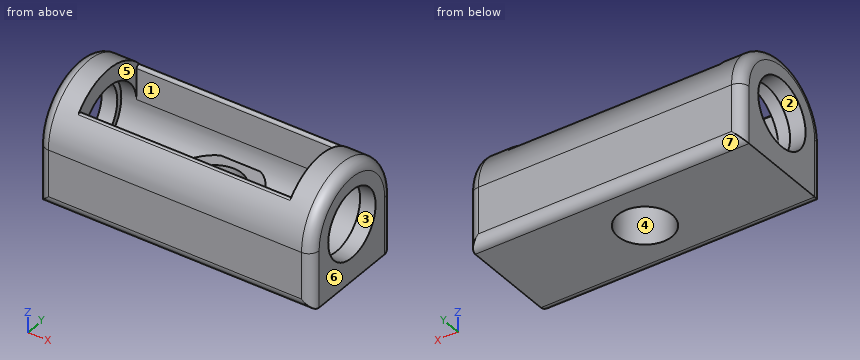
from build123d import *
from build123d.topology import SkipClean

# Parameters (mm, degrees)
BOSS_EXTRUDE1_DEPTH = 26.5
CUT_EXTRUDE2_REACH  = 38.729
CUT_EXTRUDE2_START  = -6
CUT_EXTRUDE3_REACH  = 32.729
SKETCH4_R           = 6.5
CUT_EXTRUDE6_START  = -3
SKETCH7_R           = 7.6000000000000005
CUT_EXTRUDE6_DEPTH  = 3
BOSS_EXTRUDE4_REACH = 60.236
BOSS_EXTRUDE4_START = -3
SKETCH8_R           = 7.999999999999998
CUT_EXTRUDE4_START  = -11
SKETCH5_R           = 5.2499999999999964
CUT_EXTRUDE4_DEPTH  = 8
FILLET1_R           = 2
FILLET2_R           = 0.5


with BuildPart() as part:
    # Sketch1 → Boss-Extrude1 (new body)
    with BuildSketch(Plane(origin=(0, 0, 0), x_dir=(0, 0, -1), z_dir=(1, 0, 0))):
        with BuildLine():
            Line((0, 11), (11.000000000000002, 11))
            Line((11.000000000000002, 11), (11.000000000000002, -11))
            Line((11.000000000000002, -11), (3.47e-15, -11))
            ThreePointArc((3.47e-15, -11), (-11, 1.35e-15), (0, 11))
        make_face()
    boss_extrude1 = extrude(amount=BOSS_EXTRUDE1_DEPTH)

    # Sketch3 → Cut-Extrude2 (cut, up to next)
    with BuildSketch(Plane.ZY.offset(CUT_EXTRUDE2_START), mode=Mode.PRIVATE) as cut_extrude2_sk1:
        with BuildLine():
            Line((0.7418695651929484, 7.5637047502028025), (10.999999999999998, 7.5637047502028025))
            Line((10.999999999999998, 7.5637047502028025), (11, -7.599999999999998))
            Line((11, -7.599999999999998), (9.3e-16, -7.6))
            ThreePointArc((9.3e-16, -7.6), (-7.590920764358606, 0.3713784447559566), (0.7418695651929484, 7.5637047502028025))
        make_face()
    cut_extrude2_tool1 = extrude(cut_extrude2_sk1.sketch, amount=-CUT_EXTRUDE2_REACH, mode=Mode.PRIVATE) & part.part
    cut_extrude2 = cut_extrude2_tool1.solids().sort_by_distance((6, -0.011225, 2.425795))[0]
    add(cut_extrude2, mode=Mode.SUBTRACT)

    # Sketch4 → Cut-Extrude3 (cut, up to next)
    with BuildSketch(Plane.ZY, mode=Mode.PRIVATE) as cut_extrude3_sk1:
        Circle(SKETCH4_R)
    cut_extrude3_tool1 = extrude(cut_extrude3_sk1.sketch, amount=-CUT_EXTRUDE3_REACH, mode=Mode.PRIVATE) & part.part
    cut_extrude3 = cut_extrude3_tool1.solids().sort_by_distance((0, 0, 0))[0]
    add(cut_extrude3, mode=Mode.SUBTRACT)

    # Sketch7 → Cut-Extrude6 (cut)
    with BuildSketch(Plane(origin=(6, 0, 0), x_dir=(0, 0, -1), z_dir=(1, 0, 0)).offset(CUT_EXTRUDE6_START)):
        with Locations(Location((0, 0, 0), (0, 0, 95.601814437))):
            Circle(SKETCH7_R)
    cut_extrude6 = extrude(amount=CUT_EXTRUDE6_DEPTH, mode=Mode.SUBTRACT)

    # Mirror1: Boss-Extrude1, Cut-Extrude2, Cut-Extrude3, Cut-Extrude6 across plane
    with SkipClean():  # the faces are left unmerged after this step: merging them gives an invalid solid
        add(boss_extrude1.mirror(Plane(origin=(26.5, 0, 0), x_dir=(0, 0, 1), z_dir=(1, 0, 0))))
        add(cut_extrude2.mirror(Plane(origin=(26.5, 0, 0), x_dir=(0, 0, 1), z_dir=(1, 0, 0))), mode=Mode.SUBTRACT)
        add(cut_extrude3.mirror(Plane(origin=(26.5, 0, 0), x_dir=(0, 0, 1), z_dir=(1, 0, 0))), mode=Mode.SUBTRACT)
        add(cut_extrude6.mirror(Plane(origin=(26.5, 0, 0), x_dir=(0, 0, 1), z_dir=(1, 0, 0))), mode=Mode.SUBTRACT)

    # Sketch8 → Boss-Extrude4 (add, up to next)
    with BuildSketch(Plane.XY.offset(BOSS_EXTRUDE4_START), mode=Mode.PRIVATE) as boss_extrude4_sk1:
        with Locations((26.499999999999996, 3.1e-16)):
            Circle(SKETCH8_R)
    boss_extrude4_tool1 = extrude(boss_extrude4_sk1.sketch, amount=-BOSS_EXTRUDE4_REACH, mode=Mode.PRIVATE) - part.part
    add(boss_extrude4_tool1.solids().sort_by_distance((26.5, 0, -3))[0])

    # Sketch5 → Cut-Extrude4 (cut)
    with SkipClean():  # the faces are left unmerged after this step: merging them gives an invalid solid
        with BuildSketch(Plane.XY.offset(CUT_EXTRUDE4_START)):
            with Locations((26.499999999999996, 3.1e-16)):
                Circle(SKETCH5_R)
        extrude(amount=CUT_EXTRUDE4_DEPTH, mode=Mode.SUBTRACT)

    # Fillet1
    fillet1_edges = [part.edges().sort_by_distance(p)[0] for p in [
        (53, -11, -5.500000000000003),
        (53, 11, -5.500000000000001),
        (53, -1.7e-15, 11),
        (0, -1.7e-15, 11),
        (0, 11, -5.500000000000001),
        (0, -11, -5.500000000000003),
        (26.5, 11, -11.000000000000002),
        (26.5, -11, -11.000000000000002),
    ]]
    fillet(fillet1_edges, radius=FILLET1_R)

    # Fillet2
    fillet2_edges = [part.edges().sort_by_distance(p)[0] for p in [
        (26.5, -7.599999999999999, 7.9523581408284185),
        (26.5, 7.5637047502028025, 7.9868874069789895),
    ]]
    fillet(fillet2_edges, radius=FILLET2_R)


solid = part.part
Verification items for the finished model (mm, model axes). Face numbers are marked on the shaded views. A direction names the side the tool comes from. Coordinates: 2 decimals unless noted, no trailing zeros. Write each loop counter-clockwise with the first axis right and the second up, starting at its lowest first coordinate (ties: lowest second). Pieces come first, ordered by that corner, then holes. Notation, with made-up numbers: M 74,22.25 L 99,22.25 A18 ccw 99,48.25 Z; hole C -34.75,7.25 d1. An arc over 180 degrees is marked long. One line per question, with ' | ' between items.
1) Sectioned sample at B-B on x = 5.5. Record the cut outline in (y, z).
Solutions:
outline: M -11,-9 A2 ccw -9,-11 L 9,-11 A2 ccw 11,-9 L 11,0 A11 ccw -11,0 Z; hole C 0,0 d15.2
2) Access from +Z, -Z, +X, -X, +Y, -Y to the whole of each face (thin tool, end or side, straight path). Record for the marked faces 1, 2 and 3.
Solutions:
face 1: +Z | face 2: -X | face 3: +X
3) Material ranges on L1, parallel to X at y = -0.25, z = -9; L2, parallel to Y at x = 26.5, z = -8; L3, parallel to X at y = 1.25, z = 6.75, recorded low to high.
Solutions:
L1: 0 to 21.26, 31.74 to 53 | L2: -11 to -5.25, 5.25 to 11 | L3: 0 to 3, 50 to 53
4) Sectioned sample at A-A on y = 0. State how many separate pieces and enclosed holes the cut face has, then the cut area to 3 significant figures.
Solutions:
separate pieces: 4 | enclosed holes: 0 | area: 222 mm^2
5) Depth check by flat-ended pin: pin 1 Ø3 at (x, y) = (44.5, -1.5) entering from +Z; pin 2 Ø12 at (x, z) = (40.5, 6) entering from -Y; pin 3 Ø2 at (x, y) = (44, 5) entering from +Z; pin 4 Ø4.5 at (y, z) = (-1, -1) entering from +X. Enter the tip coordinate at first touch or a pass-through.
Solutions:
pin 1: z = -6.98 | pin 2: y = -11 | pin 3: z = -4.66 | pin 4: x = 34.5
6) Release check for a two-part mould opening along X. For the marked faces 4, 5, 6 and 7 record: +X half, -X half, draft (parallel to the pull), parting line (faces both ways), or undercut.
Solutions:
face 4: undercut | face 5: undercut | face 6: +X half | face 7: draft
7) Sectioned sample at C-C on z = -5.25. Record the cut outline in (x, y).
Solutions:
outline: M 0,-9 A2 ccw 2,-11 L 51,-11 A2 ccw 53,-9 L 53,-3.83 L 50,-3.83 L 50,-5.5 L 32.31,-5.5 A8 ccw 32.31,5.5 L 50,5.5 L 50,3.83 L 53,3.83 L 53,9 A2 ccw 51,11 L 2,11 A2 ccw 0,9 L 0,3.83 L 3,3.83 L 3,5.5 L 20.69,5.5 A8 ccw 20.69,-5.5 L 3,-5.5 L 3,-3.83 L 0,-3.83 Z; hole C 26.5,0 d10.5
8) Sectioned sample at D-D on x = 26.5. Record the cut outline in (y, z).
Solutions:
outline: M -11,-9 A2 ccw -9,-11 L -5.25,-11 L -5.25,-3 L -6.98,-3 A7.6 cw -7.6,0 L -7.6,6.68 A0.5 ccw -8.49,7 A11 ccw -11,0 Z; M 5.25,-11 L 9,-11 A2 ccw 11,-9 L 11,0 A11 ccw 8.45,7.05 A0.5 ccw 7.56,6.73 L 7.56,0.74 A7.6 cw 6.98,-3 L 5.25,-3 Z
